Model file for the job. Use its own axes, mm. Coordinates: 2 decimals unless noted, no trailing zeros. Order: outer loops, then holes, each group sorted by start corner. A loop starts at its lowest first (then second) coordinate and runs counter-clockwise, first axis right, second up. Notation, with made-up numbers: M 36,-33.5 L 70,-33.5 A28 cw 70,5.5 Z; hole C 61.5,87 d11. An arc over 180 degrees is marked long. Return JSON: item names as keys, results as strings.
```python
from build123d import *

# Parameters (mm, degrees)
BOX020_W               = 24
BOX020_H               = 150
BOX020_DEPTH           = 40
BOX020_PLACEMENT_ANGLE = 15
BOX001_W               = 2
BOX001_H               = 170
BOX001_DEPTH           = 50
BOX001_PLACEMENT_ANGLE = 15


with BuildPart() as face001:
    # Box020 → Box020 (new body)
    with BuildSketch(Plane.XY):
        with Locations((12, 75)):
            Rectangle(BOX020_W, BOX020_H)
    extrude(amount=BOX020_DEPTH)


with BuildPart() as face001_1:
    # Box020 placement: moved
    add(face001.part.moved(Location((164, 10, 0))).rotate(Axis((164, 10, 0), (0, -1, 0)), BOX020_PLACEMENT_ANGLE))


with BuildPart() as cut005:
    # Box001 → Box001 (new body)
    with BuildSketch(Plane.XY):
        with Locations((1, 85)):
            Rectangle(BOX001_W, BOX001_H)
    extrude(amount=BOX001_DEPTH)


with BuildPart() as cut005_1:
    # Box001 placement: moved
    add(cut005.part.moved(Location((169, 0, -10))).rotate(Axis((169, 0, -10), (0, -1, 0)), BOX001_PLACEMENT_ANGLE))

    # Cut005: cut Face001
    add(face001_1.part, mode=Mode.SUBTRACT)


solid = cut005_1.part
```
Item 1: Drop a flat-ended pin along its axis: pin 1 Ø8 at (x, y) = (164.5, 75) entering from +Z. Give the stop position or say it passes through.
Check result:
{"pin 1": "stops at z = 1.1"}
Item 2: Saw through at C-C (y = 124). Write the cut outline in (x, z), and give its area (3 significant figures).
Check result:
{"outline": "M 166.17,0.58 L 169,-10 L 170.93,-9.48 L 168.1,1.1 Z", "area": "21.9 mm2"}
Item 3: Saw through at B-B (z = 31.5). Write the cut outline in (x, y).
Check result:
{"outline": "M 157.88,0 L 159.95,0 L 159.95,10 L 157.88,10 Z; M 157.88,160 L 159.95,160 L 159.95,170 L 157.88,170 Z"}
Item 4: Wall check: line 1 (Y direction, x = 159.25, z = 31); line 2 (X direction, y = 29, z = -5); line 3 (X direction, y = 160.5, z = -0.5). Give the ranges that are in metal, low to high.
Check result:
{"line 1": "y = 0 to 10, 160 to 170", "line 2": "x = 167.66 to 169.73", "line 3": "x = 166.45 to 168.53"}
Item 5: Pull direction Y, two halves, no side cores. Call faces 1 (the flat face through (164, 0, 14)), 2 (the flat face through (162, 10, 19)), 3 (the flat face through (166.873, 84.603, -2.063)): +Y half, -Y half, draft (parallel to the pull), parting line (faces both ways), or undercut.
Check result:
{"face 1": "-Y half", "face 2": "undercut", "face 3": "draft"}
Item 6: Saw through at A-A (x = 164.5). Write the cut outline in (y, z).
Check result:
{"outline": "M 0,6.79 L 10,6.79 L 10,14.52 L 0,14.52 Z; M 160,6.79 L 170,6.79 L 170,14.52 L 160,14.52 Z"}
